```python
from build123d import *

# Parameters (mm, degrees)
SKETCH_1_R          = 10.5
EXTRUDE_1_DEPTH     = 25
SKETCH_2_R          = 3
EXTRUDE_2_DEPTH     = 1.8
EXTRUDE_START       = -1.8
SKETCH_3_R          = 1
EXTRUDE_3_DEPTH     = 8.7
EXTRUDE_START_2     = -27.6
SKETCH_2_2_R        = 3
EXTRUDE_4_DEPTH     = 2.6
SKETCH_4_W          = 3
SKETCH_4_H          = 0.7
EXTRUDE_5_DEPTH     = 5
SKETCH_5_R          = 1.25
CUT_EXTRUDE_1_DEPTH = 5


with BuildPart() as part:
    # 草图1 → 凸台-拉伸1 (new body)
    with BuildSketch(Plane.XY):
        Circle(SKETCH_1_R)
    extrude(amount=EXTRUDE_1_DEPTH)

    # 草图2 → 凸台-拉伸2 (add)
    with BuildSketch(Plane.XY.offset(25)):
        Circle(SKETCH_2_R)
    extrude(amount=EXTRUDE_2_DEPTH)

    # 草图3 → 凸台-拉伸3 (add)
    with BuildSketch(Plane.XY.offset(26.8).offset(EXTRUDE_START)):
        Circle(SKETCH_3_R)
    extrude(amount=EXTRUDE_3_DEPTH)

    # 草图2<2> → 凸台-拉伸4 (add)
    with BuildSketch(Plane.XY.offset(25).offset(EXTRUDE_START_2)):
        Circle(SKETCH_2_2_R)
    extrude(amount=EXTRUDE_4_DEPTH)

    # 草图4 → 凸台-拉伸5 (add)
    with BuildSketch(Plane(origin=(0, 0, 0), x_dir=(-1, 0, 0), z_dir=(0, 0, -1))):
        with Locations((0, 7.85)):
            Rectangle(SKETCH_4_W, SKETCH_4_H)
        with Locations((0, -7.85)):
            Rectangle(SKETCH_4_W, SKETCH_4_H)
    extrude(amount=EXTRUDE_5_DEPTH)

    # 草图5 → 切除-拉伸1 (cut)
    with BuildSketch(Plane.XY.offset(25)):
        with Locations((0, 7.2)):
            Circle(SKETCH_5_R)
        with Locations((0, -7.2)):
            Circle(SKETCH_5_R)
    extrude(amount=-CUT_EXTRUDE_1_DEPTH, mode=Mode.SUBTRACT)


solid = part.part
```
Part model, mm, in its own coordinate system. A direction names the side the tool comes from. Coordinates: 2 decimals unless noted, no trailing zeros. Write each loop counter-clockwise with the first axis right and the second up, starting at its lowest first coordinate (ties: lowest second). Pieces come first, ordered by that corner, then holes.
Item 1: Slice it at A-A (y = 0). Write the cut outline in (x, z), and give its area (3 significant figures).
Item 2: Slice it at C-C (z = 24). Write the cut outline in (x, y).
Item 3: Probe line 1 (Y direction, x = 0, z = 21.1); line 2 (Z direction, x = 4.5, y = 6); line 3 (Z direction, x = -2.5, y = 0.75). List the from-to ranges inside material, lowest first.
Item 4: Which spindle directions (+Z, -Z, +X, -X, +Y, -Y) get a long thin tool onto all of the face, cutting with end or side? Do faces 1 (the face through (0, -8.2, -2)), 2 (the face through (0, 7.5, -2)), 3 (the face through (0, 8.2, -2)), 4 (the face through (0, -1, 30)). Say none if no direction does.
Item 5: Mould opens along X. For faces 5 (the face through (2.2, 2.5, 0)), 6 (the face through (-3, 0, -1)), 7 (the face through (-0.27, -8.42, 22.54)) say: released by +X, released by -X, zero draft, split by the parting line, or undercut.
Item 6: Pin check, flat tips, straight feed: pin 1 (0.8 mm diameter, centred on y = -8, z = -2.5, fed in from -X); pin 2 (3.5 mm diameter, centred on x = 0.5, z = -2, fed in from -Y); pin 3 (6 mm diameter, centred on x = -3.5, y = -5.5, fed in from +Z); pin 4 (10 mm diameter, centred on x = -2, z = 29.5, fed in from -Y). Stop position of each tip, or through.
Item 7: Slice it at D-D (z = 18). Write the cut outline in (x, y).
Results found:
1. outline: (-10.5, 0) - (-3, 0) - (-3, -2.6) - (3, -2.6) - (3, 0) - (10.5, 0) - (10.5, 25) - (3, 25) - (3, 26.8) - (1, 26.8) - (1, 33.7) - (-1, 33.7) - (-1, 26.8) - (-3, 26.8) - (-3, 25) - (-10.5, 25) - close
1. area: 565 mm2
2. outline: circle Ø21 at (0, 0); hole circle Ø2.5 at (0, -7.2); hole circle Ø2.5 at (0, 7.2)
3. line 1: y = -10.5 to -8.45, -5.95 to 5.95, 8.45 to 10.5
3. line 2: z = 0 to 25
3. line 3: z = -2.6 to 26.8
4. face 1: -Z, +X, -X, -Y
4. face 2: -Z, +X, -X
4. face 3: -Z, +X, -X, +Y
4. face 4: +Z
5. face 5: zero draft
5. face 6: split by the parting line
5. face 7: undercut
6. pin 1: stops at x = -1.5
6. pin 2: stops at y = -8.2
6. pin 3: stops at z = 25
6. pin 4: stops at y = -10.5
7. outline: circle Ø21 at (0, 0)
